```python
from build123d import *

# Parameters (mm, degrees)
F0_W     = 44
F0_H     = 44
F1_DEPTH = 25
F0_W_2   = 264
F0_H_2   = 264
F4_DEPTH = 50


with BuildPart() as f1:
    # F0 (on Top) → F1 (new body)
    with BuildSketch(Plane.XY):
        with Locations((-88, 0)):
            Rectangle(F0_W, F0_H)
        with Locations((-88, 88)):
            Rectangle(F0_W, F0_H)
        with Locations((0, 88)):
            Rectangle(F0_W, F0_H)
        Rectangle(F0_W, F0_H)
    extrude(amount=-F1_DEPTH)


with BuildPart() as f2_1:
    # F2: instance of F1
    add(f1.part.mirror(Plane.YZ))


with BuildPart() as f3_1:
    # F3: instance of F1
    add(f1.part.mirror(Plane.XZ))


with BuildPart() as f3_2:
    # F3: instance of F2_1
    add(f2_1.part.mirror(Plane.XZ))


with BuildPart() as f4:
    # F0 (on Top) → F4 (new body)
    with BuildSketch(Plane.XY):
        Rectangle(F0_W_2, F0_H_2)
        with Locations((-88, 0)):
            Rectangle(F0_W, F0_H, mode=Mode.SUBTRACT)
        with Locations((-88, 88)):
            Rectangle(F0_W, F0_H, mode=Mode.SUBTRACT)
        Rectangle(F0_W, F0_H, mode=Mode.SUBTRACT)
        with Locations((0, 88)):
            Rectangle(F0_W, F0_H, mode=Mode.SUBTRACT)
        with Locations((-88, 0)):
            Rectangle(F0_W, F0_H)
        Rectangle(F0_W, F0_H)
        with Locations((-88, 88)):
            Rectangle(F0_W, F0_H)
        with Locations((0, 88)):
            Rectangle(F0_W, F0_H)
    extrude(amount=-F4_DEPTH)

    # F5: cut F1, F2_1, F3_1, F3_2
    add(f1.part, mode=Mode.SUBTRACT)
    add(f2_1.part, mode=Mode.SUBTRACT)
    add(f3_1.part, mode=Mode.SUBTRACT)
    add(f3_2.part, mode=Mode.SUBTRACT)


solid = f4.part
```
Design review of the part built by this model. Coordinates are the model's own, in mm. A direction names the side the tool comes from. Coordinates: 2 decimals unless noted, no trailing zeros. Order: outer loops, then holes, each group sorted by start corner. A loop starts at its lowest first (then second) coordinate and runs counter-clockwise, first axis right, second up.
1) Take a section at A-A, the plane y = -17.5. Give the boundary of the cut face in (x, z), and give its area (3 significant figures).
2) Mouldability with a two-part tool opening along X and no side actions: class faces 1 (the flat face through (132, -2, -25)), 2 (the flat face through (0, 0, -25)), 3 (the flat face through (-2, -132, -25)) as +X half, -X half, draft (parallel to the pull), parting line (faces both ways), or undercut.
3) Take a section at C-C, the plane z = -14. State how many separate pieces and enclosed holes the cut face has, and give its area (3 significant figures).
4) For faces 4 (the flat face through (-88, 66, -12)), 5 (the flat face through (-132, -2, -25)), list the 3-axis set-ups (+Z, -Z, +X, -X, +Y, -Y) from which the entire face can be reached by the end or side of a thin tool; tool diameter is ignored.
5) Wall thickness on line 1 along X through (y, z) = (8, -18); line 2 along Z through (x, y) = (-108, 9): over which ranges is each line inside the solid? List them lowest first.
6) Clearance check with a flat-ended pin moving along its axis: pin 1 (22 mm diameter, centred on x = 86.5, y = 94.5, fed in from +Z). State where the tip first meets the part, or that it passes through.
Returned:
1. outline: (-132, -50) - (132, -50) - (132, 0) - (110, 0) - (110, -25) - (66, -25) - (66, 0) - (22, 0) - (22, -25) - (-22, -25) - (-22, 0) - (-66, 0) - (-66, -25) - (-110, -25) - (-110, 0) - (-132, 0) - close
1. area: 9,900 mm2
2. face 1: +X half
2. face 2: undercut
2. face 3: draft
3. separate pieces: 1
3. enclosed holes: 9
3. area: 52,300 mm2
4. face 4: +Z
4. face 5: +Z, -Z, -X, +Y, -Y
5. line 1: x = -132 to -110, -66 to -22, 22 to 66, 110 to 132
5. line 2: z = -50 to -25
6. pin 1: stops at z = -25
